```python
from build123d import *

# Parameters (mm, degrees)
F0_W     = 229.421454
F0_H     = 114
F1_DEPTH = 76
F3_W     = 38
F3_H     = 20
F4_DEPTH = 229.711727
F6_W     = 38
F6_H     = 38
F7_DEPTH = 114.001


with BuildPart() as f1:
    # F0 (on Front) → F1 (new body)
    with BuildSketch(Plane.XZ):
        Rectangle(F0_W, F0_H)
    extrude(amount=F1_DEPTH)

    # F3 (on offset) → F4 (cut, through all)
    with BuildSketch(Plane.YZ.offset(115)):
        with Locations((-19, 47)):
            Rectangle(F3_W, F3_H)
        with Locations((-57, -47)):
            Rectangle(F3_W, F3_H)
    extrude(amount=-F4_DEPTH, mode=Mode.SUBTRACT)

    # F6 (on offset) → F7 (cut, through all)
    with BuildSketch(Plane.XY.offset(57)):
        with Locations((-95.710727, -57)):
            Rectangle(F6_W, F6_H)
        with Locations((95.710727, -57)):
            Rectangle(F6_W, F6_H)
    extrude(amount=-F7_DEPTH, mode=Mode.SUBTRACT)


solid = f1.part
```
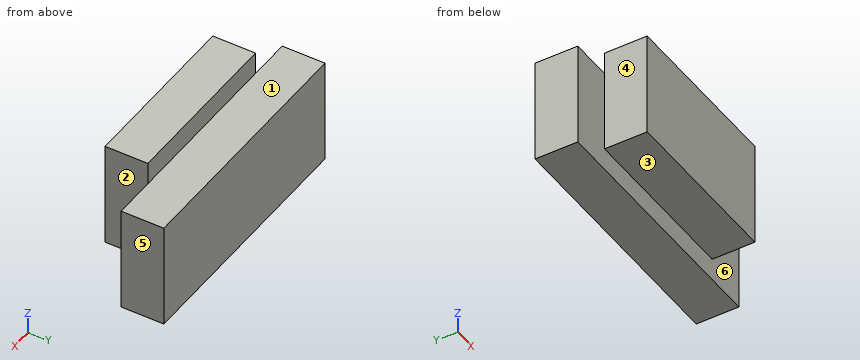
Verification items for the finished model (mm, model axes). Face numbers are marked on the shaded views. A direction names the side the tool comes from. Coordinates: 2 decimals unless noted, no trailing zeros. Loops run counter-clockwise (first coordinate to the right, second up) from the corner with the lowest first, then second, coordinate; pieces in that order, holes last. Notation, with made-up numbers: (-3, 44.25) -> (43, 44.25) arc R36 cw to (43, 78.25) -> close; hole circle Ø2 at (15, 81.25). An arc over 180 degrees is marked (long way). Put each result on its own line as item: value.
1. Section check B-B, the plane x = 31.5. Record the boundary of the cut face in (y, z), then the cut area to 3 significant figures.
Result set:
outline: (-76, -37) -> (-38, -37) -> (-38, -57) -> (0, -57) -> (0, 37) -> (-38, 37) -> (-38, 57) -> (-76, 57) -> close
area: 7,140 mm^2
2. Tool access check on the marked faces 1, 2 and 3. Record the directions out of +Z, -Z, +X, -X, +Y, -Y that give a thin tool (end or side, any length) a straight path to the whole face; none if there is none.
Result set:
face 1: +Z, +X, -X, +Y
face 2: +Z, -Z, +X, -Y
face 3: -Z, +X, -X, -Y
3. Section check C-C, the plane y = -52. Record the boundary of the cut face in (x, z), then the cut area to 3 significant figures.
Result set:
outline: (-76.71, -37) -> (76.71, -37) -> (76.71, 57) -> (-76.71, 57) -> close
area: 14,400 mm^2
4. Mould release check, pull along X, two halves, no side actions. Record for the marked faces 4, 5 and 6: pulls with the +X half, pulls with the -X half, needs draft (parallel to the pull), parting line crosses it, or undercut.
Result set:
face 4: pulls with the -X half
face 5: pulls with the +X half
face 6: needs draft
5. Section check D-D, the plane z = -41. Record the boundary of the cut face in (x, y), then the cut area to 3 significant figures.
Result set:
outline: (-114.71, -38) -> (114.71, -38) -> (114.71, 0) -> (-114.71, 0) -> close
area: 8,720 mm^2
6. Gauge pin test, flat ends, axial feed: P1, Ø19, axis at y = -63.5, z = 30.5, coming from the +X side; P2, Ø12, axis at x = -37, y = -13.5, coming from the +Z side; P3, Ø10, axis at x = -30.5, z = 42.5, coming from the +Y side. Record the tip position at first contact, or that the pin passes through.
Result set:
P1: stops at x = 76.71
P2: stops at z = 37
P3: stops at y = -38
7. Thickness scan on line 1 (Z direction, x = -20, y = -64.5); line 2 (Y direction, x = 44, z = 38.5); line 3 (Z direction, x = -37, y = -12). Record the ranges inside material, lowest first.
Result set:
line 1: z = -37 to 57
line 2: y = -76 to -38
line 3: z = -57 to 37
8. Section check A-A, the plane z = -5.5. Record the boundary of the cut face in (x, y), then the cut area to 3 significant figures.
Result set:
outline: (-114.71, -38) -> (-76.71, -38) -> (-76.71, -76) -> (76.71, -76) -> (76.71, -38) -> (114.71, -38) -> (114.71, 0) -> (-114.71, 0) -> close
area: 14,500 mm^2
